Autodesk Inventor part; units mm, degrees
ref_plane "YZ Plane" through (0, 0, 0) normal (1, 0, 0) x (0, 1, 0)
ref_plane "XZ Plane" through (0, 0, 0) normal (0, 1, 0) x (-1, 0, 0)
ref_plane "XY Plane" through (0, 0, 0) normal (0, 0, 1) x (1, 0, 0)
sketch "Sketch1" plane through (0, 0, 0) normal (0, 0, 1) x (1, 0, 0)
  circle A0 centre (0, 0) radius 11.5
  circle A1 centre (-15.5, 15.5) radius 1.5
  circle A2 centre (-15.5, -15.5) radius 1.5
  circle A3 centre (15.5, 15.5) radius 1.5
  circle A4 centre (15.5, -15.5) radius 1.5
  line L0 (-21, -24) -> (21, -24)
  line L1 (0, 20) -> (4.5462, 20) construction
  line L2 (-21, 21) -> (-1, 21)
  line L3 (1, 21) -> (21, 21)
  line L4 (-21, 21) -> (-21, 5.9161)
  line L5 (-21, -5.9161) -> (-21, -24)
  line L6 (21, 21) -> (21, 5.9161)
  line L7 (21, -5.9161) -> (21, -24)
  line L8 (-1.865, 21) -> (1.6498, 21)
  line L9 (-21, 8.451) -> (-21, -8.8551)
  line L10 (21, 10.9387) -> (21, -8.8551)
  dimension "d0" = 23
  dimension "d1" = 3
  dimension "d2" = 3
  dimension "d3" = 24
  dimension "d5" = 8.5
extrude "Extrusion1" add sketch "Sketch1" along normal blind 4
sketch "Sketch2" plane through (0, 0, 4) normal (0, 0, 1) x (1, 0, 0)
  line L0 (-21, -24) -> (21, -24)
  line L1 (21, -24) -> (21, 21)
  line L2 (-21, -24) -> (21, -24)
  line L3 (21, -24) -> (21, -18.5)
  line L4 (21, -18.5) -> (-21, -18.5)
  line L5 (-21, -18.5) -> (-21, -24)
  dimension "d9" = 5.5
extrude "Extrusion2" add sketch "Sketch2" along normal blind 10
sketch "Sketch3" plane through (-21, -24, 0) normal (0, -1, 0) x (1, 0, 0)
  line L0 (42, 0) -> (42, 14)
  line L1 (0, 0) -> (0, 14)
  circle A0 centre (5.5, 11) radius 2
  circle A1 centre (36.5, 11) radius 2
  line L2 (0, 4) -> (42, 4)
  circle A2 centre (21, 9) radius 2
  line L3 (0, 14) -> (42, 14)
  point P0 (21, 0)
  dimension "d12" = 4
  dimension "d13" = 4
  dimension "d16" = 5.5
  dimension "d17" = 5.5
  dimension "d18" = 7
  dimension "d19" = 7
  dimension "d27" = 4
  dimension "d28" = 5
sketch "Sketch4" plane through (-21, -24, 0) normal (0, -1, 0) x (1, 0, 0)
  circle A0 centre (5.5, 11) radius 2
  circle A1 centre (36.5, 11) radius 2
  arc A2 (8.1458, 14) -> (2.8542, 14) centre (5.5, 11) ccw
  arc A3 (39.1458, 14) -> (33.8542, 14) centre (36.5, 11) ccw
  line L0 (42, 14) -> (0, 14)
  line L1 (2.8542, 14) -> (8.1458, 14)
  line L2 (33.8542, 14) -> (39.1458, 14)
  point P0 (21, 0)
  dimension "d22" = 8
  dimension "d23" = 8
extrude "Extrusion4" add sketch "Sketch4" against normal blind 5.5 contours L0 A2 | A3 L0
fillet "Fillet1" radius 2 2 edges at (-21, -21.25, 14) (21, -21.25, 14)
extrude "Extrusion5" cut sketch "Sketch3" against normal blind 5.5 contours A0 | A1 | A2
sketch "Sketch5" plane through (0, 0, 0) normal (0, 0, -1) x (-1, 0, 0)
  circle A0 centre (0, 0) radius 11.5
  circle A1 centre (-15.5, -15.5) radius 1.5
  circle A2 centre (-15.5, 15.5) radius 1.5
  circle A3 centre (15.5, -15.5) radius 1.5
  circle A4 centre (15.5, 15.5) radius 1.5
  line L0 (-21, -24) -> (21, -24)
  line L1 (21, -24) -> (21, 21)
  line L2 (21, 21) -> (-21, 21)
  line L3 (-21, 21) -> (-21, -24)
extrude "Extrusion6" add sketch "Sketch5" along normal blind 4
sketch "Sketch6" plane through (-21, -18.5, 4) normal (-1, 0, 0) x (0, 0, 1)
  line L0 (-8, -5.5) -> (-8, 39.5)
  line L1 (8, -5.5) -> (-8, -5.5)
  line L2 (8, -5.5) -> (-8, -5.5)
  line L3 (-8, -5.5) -> (-8, 0)
  line L4 (-8, 0) -> (8, 0)
  line L5 (8, 0) -> (8, -5.5)
  point P0 (-4, 18.5)
extrude "Extrusion7" add sketch "Sketch6" along normal blind 30
sketch "Sketch7" plane through (21, -18.5, 4) normal (1, 0, 0) x (0, 0, -1)
  line L0 (-8, -5.5) -> (-8, 0)
  line L1 (8, -5.5) -> (-8, -5.5)
  line L2 (-8, 0) -> (8, 0)
  line L3 (8, 0) -> (8, -5.5)
  line L4 (8, -5.5) -> (-8, -5.5)
  line L5 (-8, -5.5) -> (-8, 0)
  point P0 (4, 18.5)
extrude "Extrusion8" add sketch "Sketch7" along normal blind 30
fillet "Fillet2" radius 3 2 edges at (51, -21.25, 12) (-51, -21.25, 12)
properties part number "StepperMotorPlate" material "PPS Plastic"
Input: part model. Units: mm. Frame: model coordinates. A direction names the side the tool comes from. Round coordinates to 2 decimals unless told otherwise and drop trailing zeros. Order: outer loops, then holes, each group sorted by start corner. A loop starts at its lowest first (then second) coordinate and runs counter-clockwise, first axis right, second up. Notation, with made-up numbers: (68, 57.5) - (115, 57.5) arc R12 cw to (115, 77.5) - close; hole circle Ø6 at (-14, 75). An arc over 180 degrees is marked (long way). Answer in a Markdown table with one row per item.
Item 1: Section query C-C (y = 0). Return the cut outline in (x, z), then the cut area to 3 significant figures.
Model answer:
| item | result |
|---|---|
| outline | (-21, -4) - (-11.5, -4) - (-11.5, 4) - (-21, 4) - close; (11.5, -4) - (21, -4) - (21, 4) - (11.5, 4) - close |
| area | 152 mm² |
Item 2: Section query B-B (z = -1.75). Return the cut outline in (x, y).
Model answer:
| item | result |
|---|---|
| outline | (-51, -24) - (51, -24) - (51, -18.5) - (21, -18.5) - (21, 21) - (-21, 21) - (-21, -18.5) - (-51, -18.5) - close; hole circle Ø3 at (-15.5, -15.5); hole circle Ø3 at (-15.5, 15.5); hole circle Ø23 at (0, 0); hole circle Ø3 at (15.5, -15.5); hole circle Ø3 at (15.5, 15.5) |
Item 3: Line query: line 1 (X direction, y = 15.5, z = -2.2); line 2 (Y direction, x = 15.5, z = -1.2); line 3 (X direction, y = 0, z = 3.75). Output: solid intervals per line, ascending.
Model answer:
| item | result |
|---|---|
| line 1 | x = -21 to -17, -14 to 14, 17 to 21 |
| line 2 | y = -24 to -17, -14 to 14, 17 to 21 |
| line 3 | x = -21 to -11.5, 11.5 to 21 |
Item 4: Section query D-D (z = 8). Return the cut outline in (x, y), then the cut area to 3 significant figures.
Model answer:
| item | result |
|---|---|
| outline | (-51, -24) - (-1.73, -24) - (-1.73, -18.5) - (-51, -18.5) - close; (1.73, -24) - (51, -24) - (51, -18.5) - (1.73, -18.5) - close |
| area | 542 mm² |
Item 5: Pin query (flat end, axial travel): pin 1 (4.5 mm diameter, centred on x = 39.5, y = -22, fed in from +Z); pin 2 (12 mm diameter, centred on x = -8.5, y = 11, fed in from +Z); pin 3 (5 mm diameter, centred on x = -15.5, z = 11, fed in from +Y). Return the tip coordinate at first contact, or that it passes through.
Model answer:
| item | result |
|---|---|
| pin 1 | stops at z = 12 |
| pin 2 | stops at z = 4 |
| pin 3 | stops at y = -18.5 |
Item 6: Mould query, pull axis X, two halves, no side actions, for faces 5 (the flat face through (34, -21, 12)), 6 (the flat face through (0, -21, 14)), 7 (the flat face through (51, -21, 3)). Classes: released by +X, released by -X, zero draft, split by the parting line, or undercut.
Model answer:
| item | result |
|---|---|
| face 5 | zero draft |
| face 6 | undercut |
| face 7 | released by +X |
Item 7: Section query A-A (x = -15.5). Return the cut outline in (y, z), then the cut area to 4 significant figures.
Model answer:
| item | result |
|---|---|
| outline | (-24, -4) - (-17, -4) - (-17, 4) - (-18.5, 4) - (-18.5, 9) - (-24, 9) - close; (-24, 13) - (-18.5, 13) - (-18.5, 15) - (-24, 15) - close; (-14, -4) - (14, -4) - (14, 4) - (-14, 4) - close; (17, -4) - (21, -4) - (21, 4) - (17, 4) - close |
| area | 350.5 mm² |
Item 8: Reachability of faces 1 (the flat face through (9, 10, 4)), 2 (the flat face through (-34, -21, 12)), 3 (the flat face through (-21, 1, 0)), 4 (the flat face through (-1, -18.5, 6)) from +Z, -Z, +X, -X, +Y, -Y: full face, straight path, thin tool, end or side. Return the list, or none.
Model answer:
| item | result |
|---|---|
| face 1 | +Z, +X, -X, +Y |
| face 2 | +Z, -X, +Y, -Y |
| face 3 | +Z, -Z, -X, +Y |
| face 4 | +Z, +Y |
